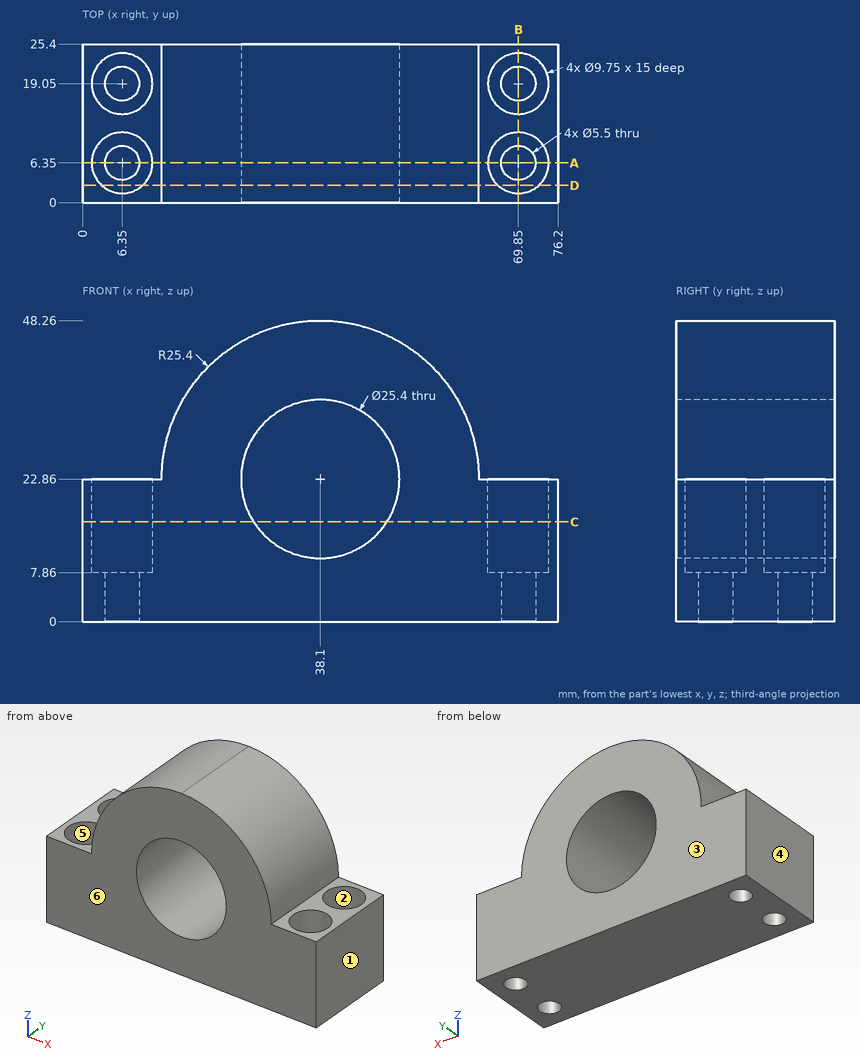
Source: three-view drawing plus pictorial views. Frame: mm from the lowest corner of the part. A direction names the side the tool comes from. Round coordinates to 2 decimals unless told otherwise and drop trailing zeros. Order: outer loops, then holes, each group sorted by start corner. A loop starts at its lowest first (then second) coordinate and runs counter-clockwise, first axis right, second up. Notation, with made-up numbers: (86, 87.25) -> (119, 87.25) arc R7 ccw to (119, 93.25) -> close; hole circle Ø9 at (-30.75, 52). An arc over 180 degrees is marked (long way). Use one line per item in the form item = value.
(1) Section A-A on y = 6.35. Return loops of the section in (x, z) (3 decimals), and give its area (3 significant figures).
Results list:
outline = (0, 0) -> (3.6, 0) -> (3.6, 7.86) -> (1.475, 7.86) -> (1.475, 22.86) -> (0, 22.86) -> close; (9.1, 0) -> (67.1, 0) -> (67.1, 7.86) -> (64.975, 7.86) -> (64.975, 22.86) -> (63.5, 22.86) arc R25.4 ccw to (12.7, 22.86) -> (11.225, 22.86) -> (11.225, 7.86) -> (9.1, 7.86) -> close; (72.6, 0) -> (76.2, 0) -> (76.2, 22.86) -> (74.725, 22.86) -> (74.725, 7.86) -> (72.6, 7.86) -> close; hole circle Ø25.4 at (38.1, 22.86)
area = 1,870 mm^2
(2) Section D-D on y = 2.75. Return loops of the section in (x, z).
Results list:
outline = (0, 0) -> (76.2, 0) -> (76.2, 22.86) -> (73.14, 22.86) -> (73.14, 7.86) -> (66.56, 7.86) -> (66.56, 22.86) -> (63.5, 22.86) arc R25.4 ccw to (12.7, 22.86) -> (9.64, 22.86) -> (9.64, 7.86) -> (3.06, 7.86) -> (3.06, 22.86) -> (0, 22.86) -> close; hole circle Ø25.4 at (38.1, 22.86)
(3) Ray query, probe 1 along Y at (x, z) = (6.35, 1.5); probe 2 along X at (y, z) = (19.25, 8); probe 3 along Y at (x, z) = (6.35, 16) (3 decimals). Return the intervals inside material, ascending. Write a range as [from, to].
Results list:
probe_1 = [0, 3.6], [9.1, 16.3], [21.8, 25.4]
probe_2 = [0, 1.48], [11.22, 64.98], [74.72, 76.2]
probe_3 = [0, 1.475], [11.225, 14.175], [23.925, 25.4]
(4) Section B-B on x = 69.85. Return loops of the section in (y, z) (3 decimals).
Results list:
outline = (0, 0) -> (3.6, 0) -> (3.6, 7.86) -> (1.475, 7.86) -> (1.475, 22.86) -> (0, 22.86) -> close; (9.1, 0) -> (16.3, 0) -> (16.3, 7.86) -> (14.175, 7.86) -> (14.175, 22.86) -> (11.225, 22.86) -> (11.225, 7.86) -> (9.1, 7.86) -> close; (21.8, 0) -> (25.4, 0) -> (25.4, 22.86) -> (23.925, 22.86) -> (23.925, 7.86) -> (21.8, 7.86) -> close
(5) Section C-C on z = 16. Return loops of the section in (x, y) (3 decimals), and give its area (3 significant figures).
Results list:
outline = (0, 0) -> (27.412, 0) -> (27.412, 25.4) -> (0, 25.4) -> close; (48.788, 0) -> (76.2, 0) -> (76.2, 25.4) -> (48.788, 25.4) -> close; hole circle Ø9.75 at (6.35, 6.35); hole circle Ø9.75 at (6.35, 19.05); hole circle Ø9.75 at (69.85, 6.35); hole circle Ø9.75 at (69.85, 19.05)
area = 1,090 mm^2
(6) Access query for the marked faces 1 and 2. Directions: +Z, -Z, +X, -X, +Y, -Y. A direction counts if a zero-diameter tool reaches every point of the face in a straight line with its end or side. Return the directions, or none.
Results list:
face_1 = +Z, -Z, +X, +Y, -Y
face_2 = +Z
(7) First-contact query: pin 1 Ø7 at (x, y) = (6.35, 6.35) entering from +Z; pin 2 Ø8 at (x, y) = (6, 20) entering from +Z; pin 3 Ø6 at (y, z) = (10, 37) entering from +X; pin 4 Ø4.5 at (x, y) = (6.35, 19.05) entering from -Z. Flat tips, straight axial feed; report the tip coordinate or a pass-through.
Results list:
pin_1 = 7.86
pin_2 = 22.86
pin_3 = 60.93
pin_4 = through
(8) Draft query along Y for the marked faces 3, 4, 5 and 6. Return one class per face: pulls with the +Y half, pulls with the -Y half, needs draft (parallel to the pull), parting line crosses it, or undercut.
Results list:
face_3 = pulls with the +Y half
face_4 = needs draft
face_5 = undercut
face_6 = pulls with the -Y half
